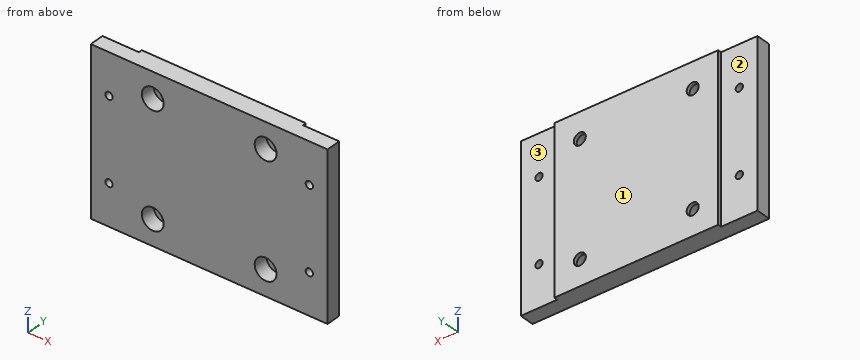
from build123d import *

# Parameters (mm, degrees)
SKETCH1_R           = 3
SKETCH1_R_2         = 1
BOSS_EXTRUDE1_DEPTH = 4
SKETCH2_W           = 45
SKETCH2_H           = 45
SKETCH2_R           = 1.65
BOSS_EXTRUDE2_DEPTH = 1


with BuildPart() as part:
    # Sketch1 → Boss-Extrude1 (new body)
    with BuildSketch(Plane(origin=(0, 0, 0), x_dir=(1, 0, 0), z_dir=(0, 1, 0))):
        Polygon((-22.5, -22.5), (-32.5, -22.5), (-32.5, 22.5), (-22.5, 22.5), (22.5, 22.5), (32.5, 22.5), (32.5, -22.5), (22.5, -22.5), align=None)
        with Locations((-15.5, 15.5)):
            Circle(SKETCH1_R, mode=Mode.SUBTRACT)
        with Locations((15.5, 15.5)):
            Circle(SKETCH1_R, mode=Mode.SUBTRACT)
        with Locations((15.5, -15.5)):
            Circle(SKETCH1_R, mode=Mode.SUBTRACT)
        with Locations((-15.5, -15.5)):
            Circle(SKETCH1_R, mode=Mode.SUBTRACT)
        with Locations((-27.5, 11.25)):
            Circle(SKETCH1_R_2, mode=Mode.SUBTRACT)
        with Locations((-27.5, -11.25)):
            Circle(SKETCH1_R_2, mode=Mode.SUBTRACT)
        with Locations((27.5, 11.25)):
            Circle(SKETCH1_R_2, mode=Mode.SUBTRACT)
        with Locations((27.5, -11.25)):
            Circle(SKETCH1_R_2, mode=Mode.SUBTRACT)
    extrude(amount=BOSS_EXTRUDE1_DEPTH)

    # Sketch2 → Boss-Extrude2 (add)
    with BuildSketch(Plane(origin=(0, 4, 0), x_dir=(1, 0, 0), z_dir=(0, 1, 0))):
        Rectangle(SKETCH2_W, SKETCH2_H)
        with Locations((-15.5, -15.5)):
            Circle(SKETCH2_R, mode=Mode.SUBTRACT)
        with Locations((15.5, -15.5)):
            Circle(SKETCH2_R, mode=Mode.SUBTRACT)
        with Locations((15.5, 15.5)):
            Circle(SKETCH2_R, mode=Mode.SUBTRACT)
        with Locations((-15.5, 15.5)):
            Circle(SKETCH2_R, mode=Mode.SUBTRACT)
    extrude(amount=BOSS_EXTRUDE2_DEPTH)


solid = part.part
Model file for the job. Use its own axes, mm. Face numbers are marked on the shaded views. A direction names the side the tool comes from. Round coordinates to 2 decimals unless told otherwise and drop trailing zeros. Order: outer loops, then holes, each group sorted by start corner. A loop starts at its lowest first (then second) coordinate and runs counter-clockwise, first axis right, second up. Notation, with made-up numbers: M 89,7 L 145,7 A38 cw 145,46 Z; hole C -39.5,28 d6. An arc over 180 degrees is marked long. Write each question's results on one line, items separated by ' | '. Start each with the question number.
(1) Saw through at B-B, the plane x = -27.5. Give the cut face in (y, z), then the cut area to 3 significant figures.
(2) Saw through at C-C, the plane y = 3.35. State how many separate pieces and enclosed holes the cut face has, then the cut area to 3 significant figures.
(3) Which spindle directions (+Z, -Z, +X, -X, +Y, -Y) get a long thin tool onto all of the face, cutting with end or side? Do the marked faces 1, 2 and 3. Say none if no direction does.
(4) Saw through at A-A, the plane z = -15.5. Give the cut face in (x, y).
(5) Probe probe 1 along Z at (x, y) = (18, 0.25); probe 2 along Z at (x, y) = (-27.5, 2.4); probe 3 along X at (y, z) = (4.4, -15.5). List the from-to ranges inside material, lowest first. Write a range as from..to.
(6) Saw through at D-D, the plane z = 8. Give the cut face in (x, y), then the cut area to 3 significant figures.
(7) Drop flat-ended pins along their axis: pin 1 (5 mm diameter, centred on x = 29.5, z = 9.5, fed in from +Y); pin 2 (4 mm diameter, centred on x = 15.5, z = 15.5, fed in from -Y); pin 3 (0.8 mm diameter, centred on y = 4.5, z = 11, fed in from +X). Give the stop position or say it passes through.
Established:
1) outline: M 0,-22.5 L 4,-22.5 L 4,-12.25 L 0,-12.25 Z; M 0,-10.25 L 4,-10.25 L 4,10.25 L 0,10.25 Z; M 0,12.25 L 4,12.25 L 4,22.5 L 0,22.5 Z | area: 164 mm^2
2) separate pieces: 1 | enclosed holes: 8 | area: 2,800 mm^2
3) face 1: +Z, -Z, +X, -X, +Y | face 2: +Z, -Z, -X, +Y | face 3: +Z, -Z, +X, +Y
4) outline: M -32.5,0 L -18.5,0 L -18.5,4 L -17.15,4 L -17.15,5 L -22.5,5 L -22.5,4 L -32.5,4 Z; M -13.85,4 L -12.5,4 L -12.5,0 L 12.5,0 L 12.5,4 L 13.85,4 L 13.85,5 L -13.85,5 Z; M 17.15,4 L 18.5,4 L 18.5,0 L 32.5,0 L 32.5,4 L 22.5,4 L 22.5,5 L 17.15,5 Z
5) probe 1: z = -22.5..-17.16, -13.84..13.84, 17.16..22.5 | probe 2: z = -22.5..-12.25, -10.25..10.25, 12.25..22.5 | probe 3: x = -22.5..-17.15, -13.85..13.85, 17.15..22.5
6) outline: M -32.5,0 L 32.5,0 L 32.5,4 L 22.5,4 L 22.5,5 L -22.5,5 L -22.5,4 L -32.5,4 Z | area: 305 mm^2
7) pin 1: stops at y = 4 | pin 2: stops at y = 4 | pin 3: stops at x = 22.5
